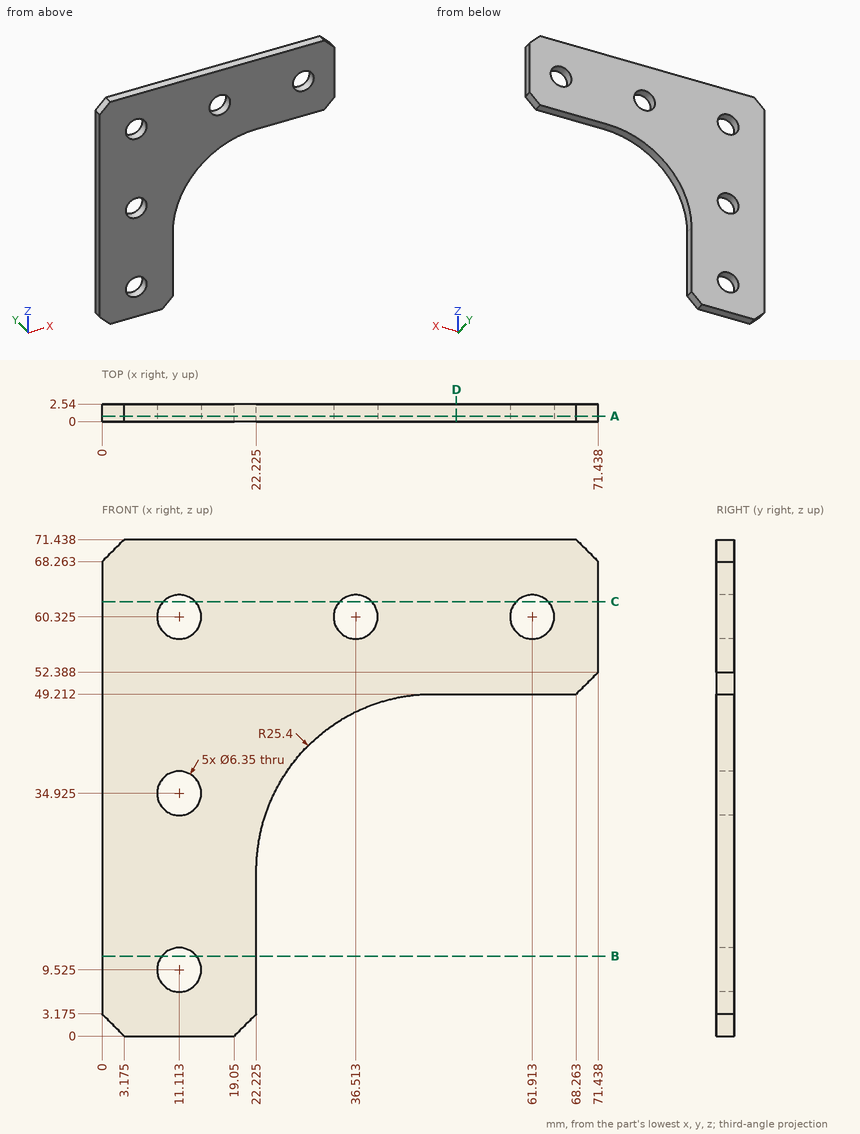
Can you work these out from the drawing? Everything is in mm from the part's minimum corner. Coordinates: 2 decimals unless noted, no trailing zeros. Write each loop counter-clockwise with the first axis right and the second up, starting at its lowest first coordinate (ties: lowest second). Pieces come first, ordered by that corner, then holes. Notation, with made-up numbers: (69, 24) -> (112, 24) arc R30 ccw to (112, 50) -> close; hole circle Ø4 at (67.5, -12). An arc over 180 degrees is marked (long way). Write each question's results on one line, items separated by ' | '. Start each with the question number.
Item 1: If we section it at A-A, the plane y = 0.8: Count the separate pieces of the cut face and the enclosed holes in it, and give its area (3 significant figures).
Item 2: Please list where these lines run through material, in increasing order: probe 1 along Z at (x, y) = (50, 0.55); probe 2 along X at (y, z) = (0.2, 12) (1 decimal); probe 3 along X at (y, z) = (0.75, 24.5) (1 decimal).
Item 3: I'm going to push flat-ended pins straight in: P1, Ø4, axis at x = 11.11, z = 9.52, coming from the -Y side; P2, Ø0.8, axis at x = 54.5, y = 1.5, coming from the -Z side. Where does each tip first touch, or does it pass through?
Item 4: If we section it at D-D, the plane x = 51: Write out the boundary of the cut face in (y, z).
Item 5: If we section it at B-B, the plane z = 11.5: Write out the boundary of the cut face in (x, y) (1 decimal).
Item 6: If we section it at C-C, the plane z = 62.5: Write out the boundary of the cut face in (x, y) (1 decimal), and give its area (3 significant figures).
Answer block:
1) separate pieces: 1 | enclosed holes: 5 | area: 2,640 mm²
2) probe 1: 49.21 to 71.44 | probe 2: 0 to 9.1, 13.1 to 22.2 | probe 3: 0 to 22.2
3) P1: through | P2: z = 49.21
4) outline: (0, 49.21) -> (2.54, 49.21) -> (2.54, 71.44) -> (0, 71.44) -> close
5) outline: (0, 0) -> (8.6, 0) -> (8.6, 2.5) -> (0, 2.5) -> close; (13.6, 0) -> (22.2, 0) -> (22.2, 2.5) -> (13.6, 2.5) -> close
6) outline: (0, 0) -> (8.8, 0) -> (8.8, 2.5) -> (0, 2.5) -> close; (13.4, 0) -> (34.2, 0) -> (34.2, 2.5) -> (13.4, 2.5) -> close; (38.8, 0) -> (59.6, 0) -> (59.6, 2.5) -> (38.8, 2.5) -> close; (64.2, 0) -> (71.4, 0) -> (71.4, 2.5) -> (64.2, 2.5) -> close | area: 146 mm²
